from build123d import *

# Parameters (mm, degrees)
F0_W     = 33.333
F0_H     = 166.666
F2_W     = 89.51439
F2_H     = 89.51439
F3_DEPTH = 10


with BuildPart() as f1:
    # F0 (on Front) → F1 (revolve)
    with BuildSketch(Plane.XZ):
        with Locations((16.6665, 83.333)):
            Rectangle(F0_W, F0_H)
    revolve(axis=Axis((0, 0, 83.333), (0, 0, -1)))

    # F2 (on Top) → F3 (join)
    with BuildSketch(Plane.XY):
        Rectangle(F2_W, F2_H)
    extrude(amount=F3_DEPTH)


solid = f1.part
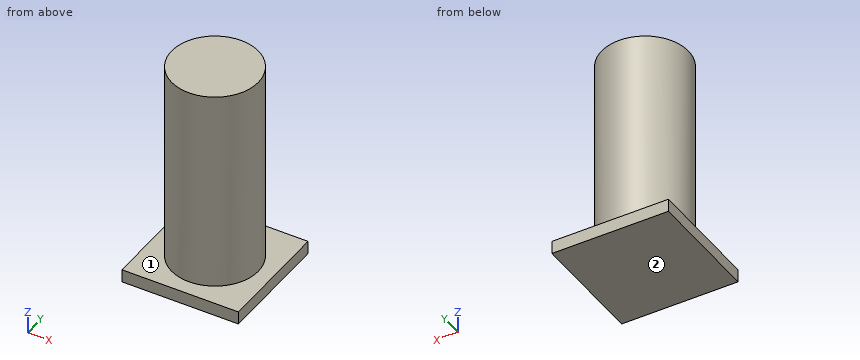
Read the model definition and answer for the solid it produces. Units are mm, in the model's axes. Face numbers are marked on the shaded views. A direction names the side the tool comes from. Coordinates: 2 decimals unless noted, no trailing zeros. Loops run counter-clockwise (first coordinate to the right, second up) from the corner with the lowest first, then second, coordinate; pieces in that order, holes last. Notation, with made-up numbers: (39.5, 36.25) -> (44.5, 36.25) arc R9 ccw to (44.5, 49.25) -> close; hole circle Ø8 at (-32, -14). An arc over 180 degrees is marked (long way). Write item = value, one per line. Start each with the question number.
1) The part is cut by section A-A, the plane x = 0. Determine the outline of the cut face in (y, z).
2) The part is cut by section C-C, the plane z = 133. Determine the outline of the cut face in (x, y), plus the area to 3 significant figures.
3) Find the intervals of material crossed by L1, parallel to Z at x = -15.5, y = -31; L2, parallel to Y at x = 1.5, z = 140, in increasing order. Write a range as from..to.
4) The part is cut by section D-D, the plane y = 35.5. Determine the outline of the cut face in (x, z).
5) Given P1, Ø12, axis at y = 11.5, z = 60, coming from the -X side; P2, Ø5, axis at x = 0.5, z = 19.5, coming from the -Y side; P3, Ø8, axis at x = 6.5, z = 30, coming from the +Y side, each flat-ended and moving along its own axis, determine where each tip first touches the part or whether it passes through.
6) For the marked faces 1 and 2, determine the directions among +Z, -Z, +X, -X, +Y, -Y from which every point of the face is accessible in a straight line to the end or side of a thin tool.
Result:
q1.outline = (-44.76, 0) -> (44.76, 0) -> (44.76, 10) -> (33.33, 10) -> (33.33, 166.67) -> (-33.33, 166.67) -> (-33.33, 10) -> (-44.76, 10) -> close
q2.outline = circle Ø66.67 at (0, 0)
q2.area = 3,490 mm²
q3.L1 = 0..10
q3.L2 = -33.3..33.3
q4.outline = (-44.76, 0) -> (44.76, 0) -> (44.76, 10) -> (-44.76, 10) -> close
q5.P1 = -32.88
q5.P2 = -33.33
q5.P3 = 33.24
q6.face_1 = +Z
q6.face_2 = -Z, +X, -X, +Y, -Y
